For this review, use the dimensioned drawing (mm, ordinates from the lowest corner) and the shaded views. A direction names the side the tool comes from. Round coordinates to 2 decimals unless told otherwise and drop trailing zeros. Write each loop counter-clockwise with the first axis right and the second up, starting at its lowest first coordinate (ties: lowest second). Pieces come first, ordered by that corner, then holes. Notation, with made-up numbers: (-17.75, 1.25) -> (7.25, 1.25) arc R10 ccw to (7.25, 12.25) -> close; hole circle Ø4 at (-3, 40.5). An arc over 180 degrees is marked (long way). Answer as CSV lines item,"result". Start each with the question number.
Item 1: Machinability: for the marked faces 4 and 5, which of the approach directions +Z, -Z, +X, -X, +Y, -Y give a long, thin tool a straight path to every point of the face, cutting with its end or side? Answer none if there is none.
Item 2: For pin 1 Ø4.5 at (x, z) = (4.56, 20) entering from -Y; pin 2 Ø5 at (x, y) = (25, 41) entering from -Z; pin 3 Ø6 at (x, z) = (31.5, 23) entering from -Y, all flat-tipped, find the tip position at first contact; note any pin that passes through.
Item 3: Take a section at C-C on x = 22.5. Give the boundary of the cut face in (y, z).
Item 4: Take a section at B-B on y = 53.5. Give the boundary of the cut face in (x, z).
Item 5: Take a section at A-A on z = 20. Give the boundary of the cut face in (x, y).
Item 6: Take a section at D-D on x = 4. Give the boundary of the cut face in (y, z).
Item 7: Mouldability with a two-part tool opening along Z and no side actions: class the marked faces 1, 2 and 3 as +Z half, -Z half, draft (parallel to the pull), parting line (faces both ways), or undercut.
Item 8: Wall thickness on probe 1 along X at (y, z) = (58.95, 20); probe 2 along Z at (x, y) = (11, 22); probe 3 along Y at (x, z) = (22.5, 0.35): over which ranges is each line inside the solid? List them lowest first. Write a range as from..to.
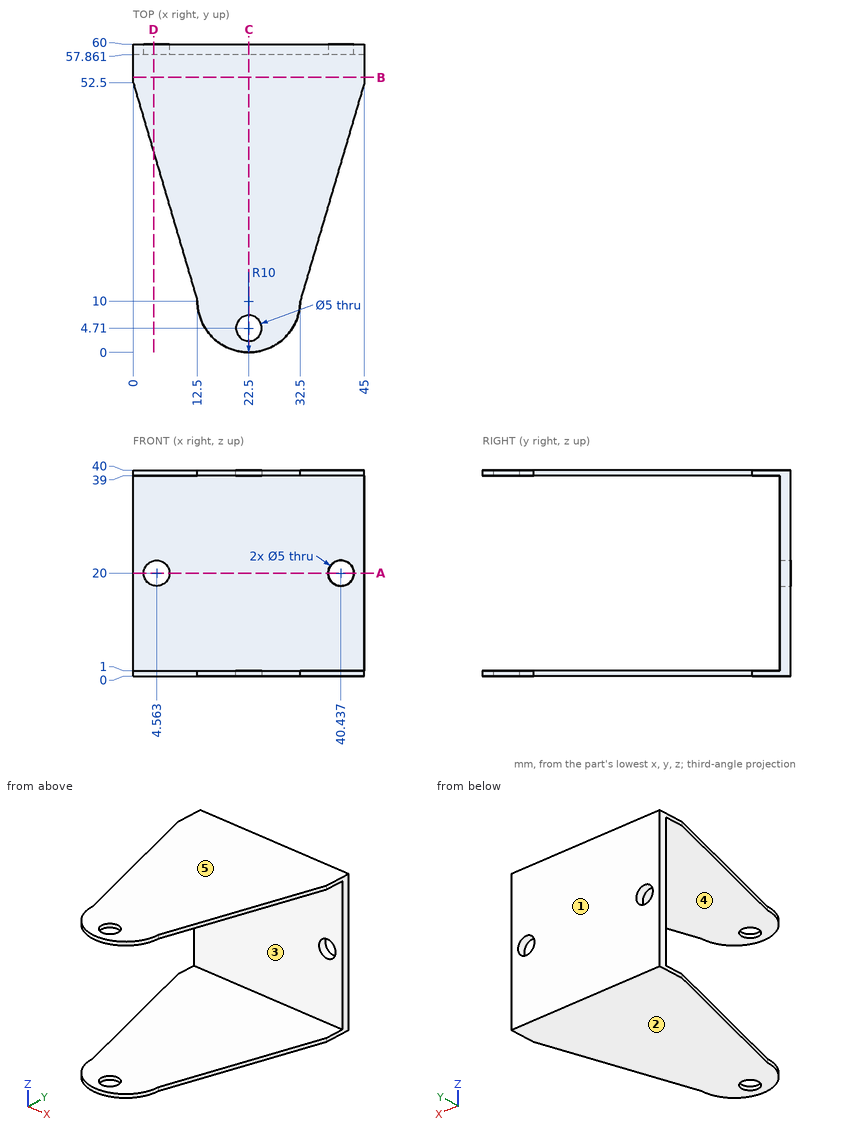
Output values:
1,face 4,"+X, -X, -Y"
1,face 5,"+Z, +X, -X, +Y, -Y"
2,pin 1,"passes through"
2,pin 2,"stops at z = 0"
2,pin 3,"stops at y = 57.86"
3,outline,"(0, 0) -> (2.21, 0) -> (2.21, 1) -> (0, 1) -> close; (0, 39) -> (2.21, 39) -> (2.21, 40) -> (0, 40) -> close; (7.21, 0) -> (60, 0) -> (60, 40) -> (7.21, 40) -> (7.21, 39) -> (57.86, 39) -> (57.86, 1) -> (7.21, 1) -> close"
4,outline,"(0, 0) -> (45, 0) -> (45, 1) -> (0, 1) -> close; (0, 39) -> (45, 39) -> (45, 40) -> (0, 40) -> close"
5,outline,"(0, 57.86) -> (2.06, 57.86) -> (2.06, 60) -> (0, 60) -> close; (7.06, 57.86) -> (37.94, 57.86) -> (37.94, 60) -> (7.06, 60) -> close; (42.94, 57.86) -> (45, 57.86) -> (45, 60) -> (42.94, 60) -> close"
6,outline,"(38.9, 0) -> (60, 0) -> (60, 17.56) -> (57.86, 17.56) -> (57.86, 1) -> (38.9, 1) -> close; (38.9, 39) -> (57.86, 39) -> (57.86, 22.44) -> (60, 22.44) -> (60, 40) -> (38.9, 40) -> close"
7,face 1,"draft"
7,face 2,"-Z half"
7,face 3,"undercut"
8,probe 1,"x = 0..2.06, 7.06..37.94, 42.94..45"
8,probe 2,"z = 0..1, 39..40"
8,probe 3,"y = 0..2.21, 7.21..60"
